Build history of the part. All positions in model axes, mm. A direction names the side the tool comes from. Give positions to 0.01 mm unless a question says otherwise; leave off trailing zeros. Order: outer loops, then holes, each group sorted by start corner. A loop starts at its lowest first (then second) coordinate and runs counter-clockwise, first axis right, second up. Notation, with made-up numbers: (25, -22) -> (67, -22) arc R22 ccw to (67, -2) -> close; hole circle Ø4 at (61, 2). An arc over 180 degrees is marked (long way). Use a Markdown table: item, result. Add a question column.
```python
from build123d import *

# Parameters (mm, degrees)
BOSS_EXTRUDE1_DEPTH = 19
SKETCH2_R           = 2.75
CUT_EXTRUDE1_DEPTH  = 21
SKETCH3_R           = 2.75
CUT_EXTRUDE2_DEPTH  = 21


with BuildPart() as part:
    # Sketch1 → Boss-Extrude1 (new body, symmetric)
    with BuildSketch(Plane.XY):
        with BuildLine():
            Line((0, 0), (0, 20))
            ThreePointArc((0, 20), (2.121320344, 19.121320344), (3, 17))
            Line((3, 17), (3, 6))
            ThreePointArc((3, 6), (3.878679656, 3.878679656), (6, 3))
            Line((6, 3), (17, 3))
            ThreePointArc((17, 3), (19.121320344, 2.121320344), (20, 0))
            Line((20, 0), (0, 0))
        make_face()
    extrude(amount=BOSS_EXTRUDE1_DEPTH, both=True)

    # Sketch2 → Cut-Extrude1 (cut, through all)
    with BuildSketch(Plane(origin=(0, 0, 0), x_dir=(1, 0, 0), z_dir=(0, 1, 0))):
        with Locations((10, -10)):
            Circle(SKETCH2_R)
        with Locations((10, 10)):
            Circle(SKETCH2_R)
    extrude(amount=CUT_EXTRUDE1_DEPTH, mode=Mode.SUBTRACT)

    # Sketch3 → Cut-Extrude2 (cut, through all)
    with BuildSketch(Plane(origin=(0, 0, 0), x_dir=(0, 0, -1), z_dir=(1, 0, 0))):
        with Locations((-10, 10)):
            Circle(SKETCH3_R)
        with Locations((10, 10)):
            Circle(SKETCH3_R)
    extrude(amount=CUT_EXTRUDE2_DEPTH, mode=Mode.SUBTRACT)


solid = part.part
```
(1) Wall check: probe 1 along Z at (x, y) = (10, 0.85); probe 2 along Z at (x, y) = (2.5, 7.75); probe 3 along X at (y, z) = (11.25, -7). Give the ranges that are in metal, low to high.
(2) Mould opens along Z. For faces 1 (the face through (11.48, 1.48, -12.32)), 2 (the face through (4, 3, 19)), 3 (the face through (2.1, 19.14, 0.27)) say: released by +Z, released by -Z, zero draft, split by the parting line, or undercut.
(3) Band-saw the part on D-D on z = -15. Give the cut face in (x, y).
(4) Band-saw the part on A-A on x = 10. Give the cut face in (y, z), plus the area to 3 significant figures.
(5) Pin check, flat tips, straight feed: pin 1 Ø9 at (y, z) = (9, 1) entering from +X; pin 2 Ø3.5 at (x, z) = (11.5, 8) entering from +Y. Stop position of each tip, or through.
(6) Band-saw the part on C-C on z = -10. Give the cut face in (x, y), plus the area to 3 significant figures.
(7) Tool access for faces 4 (the face through (1.48, 12.32, -11.48)), 5 (the face through (3, 12, 0)): list every direction of +Z, -Z, +X, -X, +Y, -Y with a clear straight run to the whole face (end or side of a thin tool).
Response:
| question | item | result |
|---|---|---|
| 1 | probe 1 | z = -19 to -12.75, -7.25 to 7.25, 12.75 to 19 |
| 1 | probe 2 | z = -19 to -11.58, -8.42 to 8.42, 11.58 to 19 |
| 1 | probe 3 | x = 0 to 3 |
| 2 | face 1 | undercut |
| 2 | face 2 | released by +Z |
| 2 | face 3 | zero draft |
| 3 | outline | (0, 0) -> (20, 0) arc R3 ccw to (17, 3) -> (6, 3) arc R3 cw to (3, 6) -> (3, 17) arc R3 ccw to (0, 20) -> close |
| 4 | outline | (0, -19) -> (3, -19) -> (3, -12.75) -> (0, -12.75) -> close; (0, -7.25) -> (3, -7.25) -> (3, 7.25) -> (0, 7.25) -> close; (0, 12.75) -> (3, 12.75) -> (3, 19) -> (0, 19) -> close |
| 4 | area | 81.0 mm² |
| 5 | pin 1 | stops at x = 3.4 |
| 5 | pin 2 | stops at y = 3 |
| 6 | outline | (0, 0) -> (7.25, 0) -> (7.25, 3) -> (6, 3) arc R3 cw to (3, 6) -> (3, 7.25) -> (0, 7.25) -> close; (0, 12.75) -> (3, 12.75) -> (3, 17) arc R3 ccw to (0, 20) -> close; (12.75, 0) -> (20, 0) arc R3 ccw to (17, 3) -> (12.75, 3) -> close |
| 6 | area | 76.1 mm² |
| 7 | face 4 | +X, -X |
| 7 | face 5 | +Z, -Z, +X, +Y |
